Could you check a few things on this model? Use its own coordinates, in mm. Round coordinates to 2 decimals unless told otherwise and drop trailing zeros. Write each loop counter-clockwise with the first axis right and the second up, starting at its lowest first coordinate (ties: lowest second). Pieces come first, ordered by that corner, then holes. Notation, with made-up numbers: (-11, 48.5) -> (3, 48.5) arc R31 cw to (3, 87.5) -> close; hole circle Ø3 at (71.25, 57). An arc over 180 degrees is marked (long way). Answer in a Markdown table with one row per item.
from build123d import *

# Parameters (mm, degrees)
F1_DEPTH = 12


with BuildPart() as f1:
    # F0 (on Top) → F1 (new body)
    with BuildSketch(Plane.XY):
        with BuildLine():
            Line((290, 149.358979), (0, 149.358979))
            Line((0, 149.358979), (0, 1.5))
            ThreePointArc((0, 1.5), (1.06066, 1.06066), (1.5, 0))
            ThreePointArc((1.5, 0), (1.06066, -1.06066), (0, -1.5))
            Line((0, -1.5), (0, -150.641021))
            Line((0, -150.641021), (290, -150.641021))
            Line((290, -150.641021), (290, 149.358979))
        make_face()
        with BuildLine():
            ThreePointArc((240, -4.5), (235.5, 0), (240, 4.5))
            Line((240, 4.5), (248.606404, 4.5))
            ThreePointArc((248.606404, 4.5), (267.270337, 16.847717), (282, 0))
            ThreePointArc((282, 0), (267.270337, -16.847717), (248.606404, -4.5))
            Line((248.606404, -4.5), (240, -4.5))
        make_face(mode=Mode.SUBTRACT)
        with BuildLine():
            Line((0, 1.5), (0, 149.358979))
            Line((0, 149.358979), (-290, 149.358979))
            Line((-290, 149.358979), (-290, -150.641021))
            Line((-290, -150.641021), (0, -150.641021))
            Line((0, -150.641021), (0, -1.5))
            ThreePointArc((0, -1.5), (-1.5, 0), (0, 1.5))
        make_face()
        with BuildLine():
            ThreePointArc((-240, 4.5), (-236.818019, 3.181981), (-235.5, 0))
            ThreePointArc((-235.5, 0), (-236.818019, -3.181981), (-240, -4.5))
            Line((-240, -4.5), (-248.606404, -4.5))
            ThreePointArc((-248.606404, -4.5), (-282, 0), (-248.606404, 4.5))
            Line((-248.606404, 4.5), (-240, 4.5))
        make_face(mode=Mode.SUBTRACT)
    extrude(amount=F1_DEPTH)


solid = f1.part
1) Please list where these lines run through material, in increasing order: line 1 (Y direction, x = -265, z = 5.5); line 2 (Y direction, x = -245, z = 2.25).
Findings:
| item | result |
|---|---|
| line 1 | y = -150.64 to -17, 17 to 149.36 |
| line 2 | y = -150.64 to -4.5, 4.5 to 149.36 |
2) Thinking about a two-plate mould opening in X: for faces 1 (the face through (-4, -150.641, 6)), 2 (the face through (-281.986, -0.684, 5.916)), 3 (the face through (290, -3, 6)), which applies, +X half, -X half, draft (parallel to the pull), parting line (faces both ways), or undercut?
Findings:
| item | result |
|---|---|
| face 1 | draft |
| face 2 | undercut |
| face 3 | +X half |
3) Imagine slicing it at A-A, the plane x = -265. Please give me the cut outline in (y, z).
Findings:
| item | result |
|---|---|
| outline | (-150.64, 0) -> (-17, 0) -> (-17, 12) -> (-150.64, 12) -> close; (17, 0) -> (149.36, 0) -> (149.36, 12) -> (17, 12) -> close |
